The figure shows three views and two pictorial views of one solid part (mm, origin at its lowest corner). Answer the questions. Give positions to 0.01 mm unless a question says otherwise; leave off trailing zeros. Loops run counter-clockwise (first coordinate to the right, second up) from the corner with the lowest first, then second, coordinate; pieces in that order, holes last. Notation, with made-up numbers: (82, 81) - (117, 81) arc R22 ccw to (117, 103) - close; hole circle Ø11 at (73.5, 66.5). An arc over 180 degrees is marked (long way). Use a Markdown table: item, result. Add a question column.
Item 1: A cutting plane is placed at C-C (y = 3.5). Determine the outline of the cut face in (x, z).
Item 2: A cutting plane is placed at D-D (x = 30). Determine the outline of the cut face in (y, z), plus the area to 3 significant figures.
Item 3: A cutting plane is placed at B-B (y = 56.5). Determine the outline of the cut face in (x, z), plus the area to 3 significant figures.
Item 4: This flat-tipped pin is pushed along its axis until it touches: P1, Ø1.8, axis at x = 32.5, z = 2, coming from the +Y side. Where does it stop, or does it pass through?
Item 5: A cutting plane is placed at A-A (z = 2). Give the number of separate pieces and of enclosed holes in the cut face, plus the area to 3 significant figures.
Item 6: Consider probe 1 along X at (y, z) = (64, 3.35); probe 2 along X at (y, z) = (3.5, 1.45); probe 3 along X at (y, z) = (4.5, 3.25) (1 decimal). Determine where each line is inside the solid, lowest interval first. Write a range as [from, to].
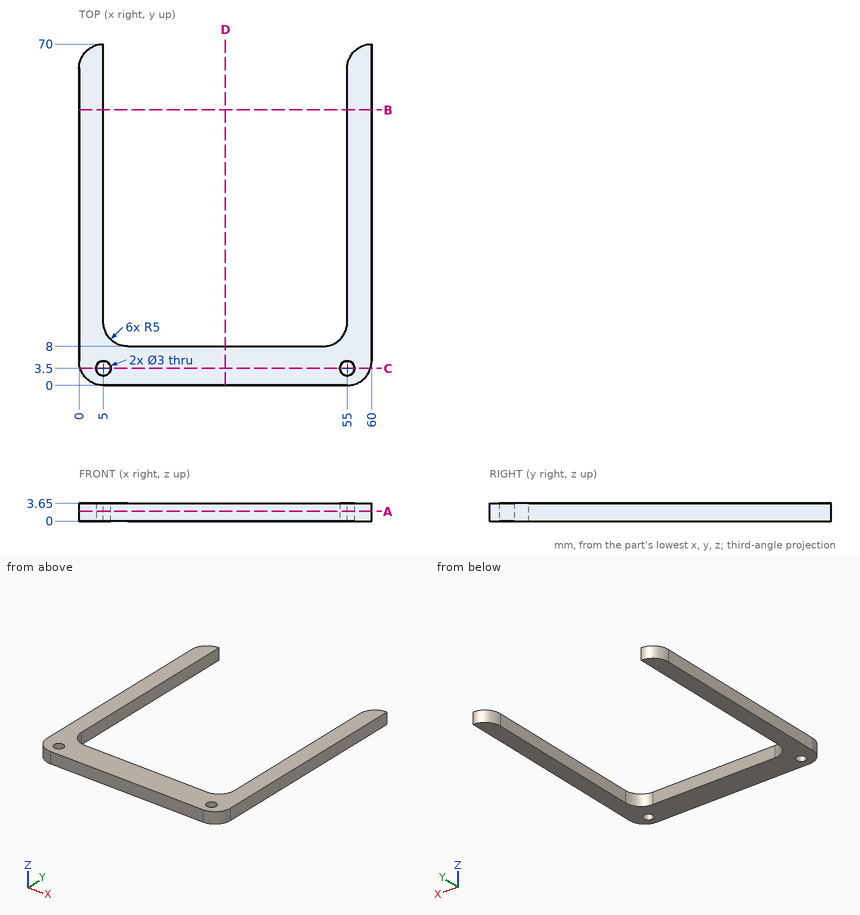
Geometry says:
| question | item | result |
|---|---|---|
| 1 | outline | (0.23, 0) - (3.5, 0) - (3.5, 3.65) - (0.23, 3.65) - close; (6.5, 0) - (53.5, 0) - (53.5, 3.65) - (6.5, 3.65) - close; (56.5, 0) - (59.77, 0) - (59.77, 3.65) - (56.5, 3.65) - close |
| 2 | outline | (0, 0) - (8, 0) - (8, 3.65) - (0, 3.65) - close |
| 2 | area | 29.2 mm² |
| 3 | outline | (0, 0) - (5, 0) - (5, 3.65) - (0, 3.65) - close; (55, 0) - (60, 0) - (60, 3.65) - (55, 3.65) - close |
| 3 | area | 36.5 mm² |
| 4 | P1 | y = 8 |
| 5 | separate pieces | 1 |
| 5 | enclosed holes | 2 |
| 5 | area | 1,080 mm² |
| 6 | probe 1 | [0, 5], [55, 60] |
| 6 | probe 2 | [0.23, 3.5], [6.5, 53.5], [56.5, 59.77] |
| 6 | probe 3 | [0, 3.9], [6.1, 53.9], [56.1, 60] |
